Input: dimensioned drawing with shaded views. Units: mm. Origin: part minimum x, y, z. A direction names the side the tool comes from. Give positions to 0.01 mm unless a question says otherwise; leave off trailing zeros. Write each loop counter-clockwise with the first axis right and the second up, starting at its lowest first coordinate (ties: lowest second). Pieces come first, ordered by that corner, then holes.
Q1. Section D-D (z = 21.5). Return the cut outline in (x, y).
Q2. Section A-A (z = 7). Return the cut outline in (x, y).
Q3. Section C-C (x = 12). Return the cut outline in (y, z), plus the area to 3 significant figures.
Q4. Reachability of the marked faces 1 and 2 from +Z, -Z, +X, -X, +Y, -Y: full face, straight path, thin tool, end or side. Return the list, or none.
Q5. Pin query (flat end, axial travel): pin 1 Ø2.5 at (x, y) = (12.5, 11) entering from -Z; pin 2 Ø2 at (y, z) = (7.5, 17.5) entering from +X; pin 3 Ø9 at (x, y) = (12, 10) entering from +Z; pin 4 Ø4 at (x, z) = (8, 22.5) entering from +Y. Return the tip coordinate at first contact, or that it passes through.
Q6. Section B-B (y = 15.5). Return the cut outline in (x, z), plus the area to 3 significant figures.
Q7. Line query: line 1 (X direction, y = 10, z = 33.05); line 2 (X direction, y = 10, z = 30.6); line 3 (Z direction, x = 4.55, y = 10). Output: solid intervals per line, ascending.
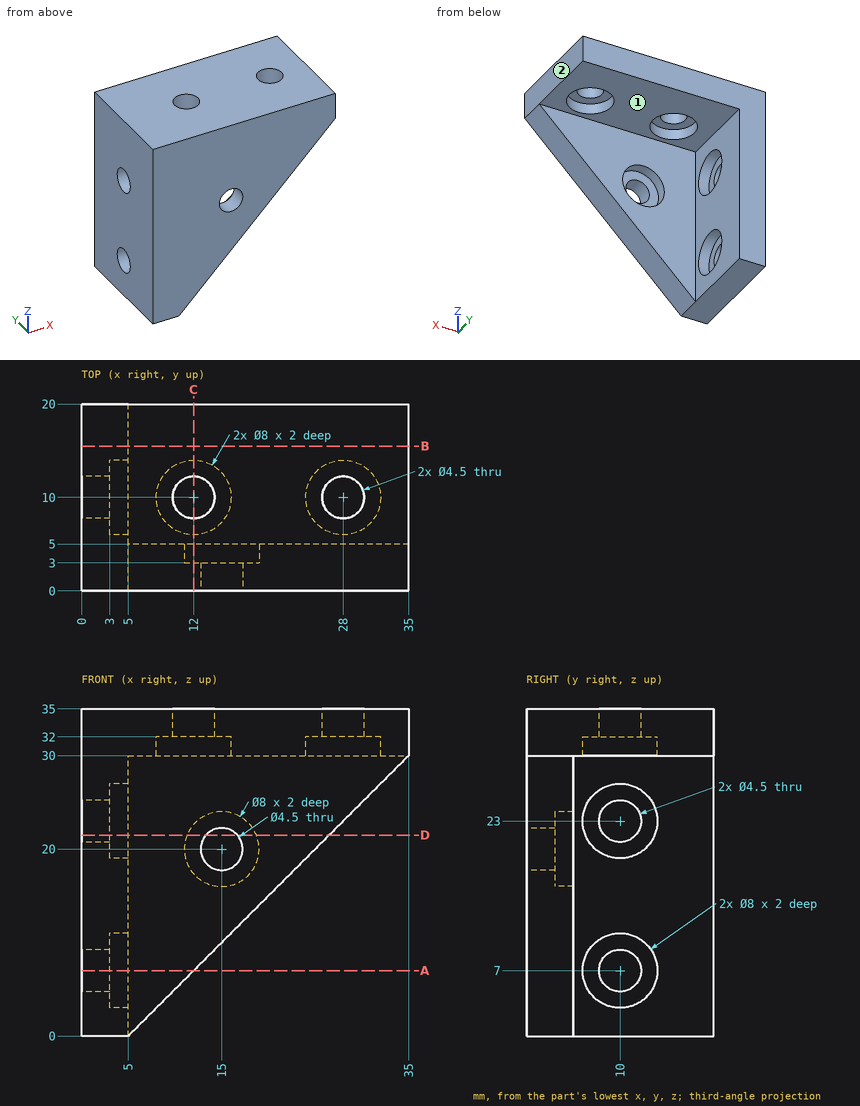
Computed:
1. outline: (0, 0) - (13.32, 0) - (13.32, 3) - (11.29, 3) - (11.29, 5) - (5, 5) - (5, 6.29) - (3, 6.29) - (3, 8.32) - (0, 8.32) - close; (0, 11.68) - (3, 11.68) - (3, 13.71) - (5, 13.71) - (5, 20) - (0, 20) - close; (16.68, 0) - (26.5, 0) - (26.5, 5) - (18.71, 5) - (18.71, 3) - (16.68, 3) - close
2. outline: (0, 0) - (12, 0) - (12, 5) - (5, 5) - (5, 6) - (3, 6) - (3, 7.75) - (0, 7.75) - close; (0, 12.25) - (3, 12.25) - (3, 14) - (5, 14) - (5, 20) - (0, 20) - close
3. outline: (0, 7) - (5, 7) - (5, 17.35) - (3, 17.35) - (3, 22.65) - (5, 22.65) - (5, 30) - (6, 30) - (6, 32) - (7.75, 32) - (7.75, 35) - (0, 35) - close; (12.25, 32) - (14, 32) - (14, 30) - (20, 30) - (20, 35) - (12.25, 35) - close
3. area: 175 mm2
4. face 1: -Z, +X, +Y
4. face 2: +Z, -Z, +X, +Y, -Y
5. pin 1: stops at z = 32
5. pin 2: stops at x = 5
5. pin 3: stops at z = 35
5. pin 4: stops at y = 5
6. outline: (0, 0) - (5, 0) - (5, 30) - (35, 30) - (35, 35) - (0, 35) - close
6. area: 325 mm2
7. line 1: x = 0 to 9.75, 14.25 to 25.75, 30.25 to 35
7. line 2: x = 0 to 8, 16 to 24, 32 to 35
7. line 3: z = 0 to 3, 11 to 19, 27 to 35
